Geometry: final body of the model. Coordinates: model frame, mm. Face numbers are marked on the shaded views. A direction names the side the tool comes from. Give positions to 0.01 mm unless a question says otherwise; leave off trailing zeros. Order: outer loops, then holes, each group sorted by start corner. A loop starts at its lowest first (then second) coordinate and runs counter-clockwise, first axis right, second up. Notation, with made-up numbers: (58.5, 21.25) - (83.5, 21.25) arc R19 ccw to (83.5, 57.25) - close; hole circle Ø5 at (66, -21). An arc over 180 degrees is marked (long way). Use one line per item in the form item = value.
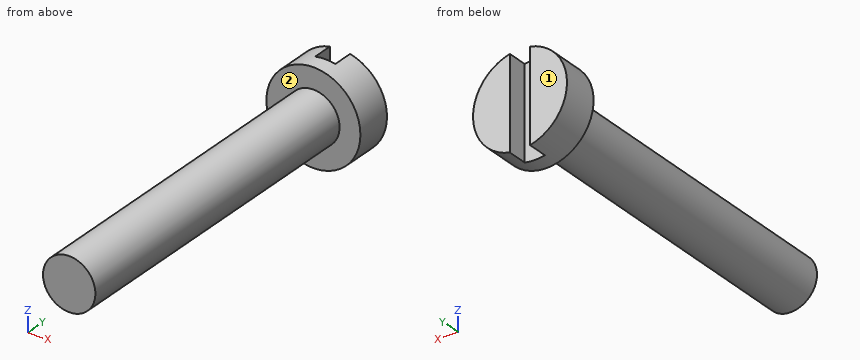
Autodesk Inventor part; units mm, degrees
ref_plane "YZ Plane" through (0, 0, 0) normal (1, 0, 0) x (0, 1, 0)
ref_plane "XZ Plane" through (0, 0, 0) normal (0, 1, 0) x (-1, 0, 0)
ref_plane "XY Plane" through (0, 0, 0) normal (0, 0, 1) x (1, 0, 0)
sketch "Sketch1" plane through (0, 0, 0) normal (0, 1, 0) x (-1, 0, 0)
  circle A0 centre (0, 0) radius 1.95
  dimension "d0" = 3.9
extrude "Extrusion1" add sketch "Sketch1" along normal blind 24.8
sketch "Sketch2" plane through (0, 24.8, 0) normal (0, 1, 0) x (1, 0, 0)
  circle A0 centre (0, 0) radius 3.5
  dimension "d3" = 7
extrude "Extrusion2" add sketch "Sketch2" along normal blind 2.7
sketch "Sketch3" plane through (0, 27.5, 0) normal (0, 1, 0) x (1, 0, 0)
  line L0 (0.75, -8) -> (-0.75, -8)
  line L1 (-0.75, -8) -> (-0.75, 8)
  line L2 (-0.75, 8) -> (0.75, 8)
  line L3 (0.75, 8) -> (0.75, -8)
  line L4 (0.75, -8) -> (-0.75, 8) construction
  line L5 (-0.75, -8) -> (0.75, 8) construction
  point P0 (0, 0)
  dimension "d6" = 1.5
  dimension "d7" = 16
extrude "Extrusion3" cut sketch "Sketch3" against normal blind 1.5
properties part number "screw27x4mm" material "Stainless Steel"
(1) Cut plane C-C on y = 20. Output: boundary loops of the cut face in (x, z), plus the area to 3 significant figures.
Computed values:
outline = circle Ø3.9 at (0, 0)
area = 11.9 mm²
(2) Contact query for flat-ended pins moving along their axis: pin 1 Ø3 at (x, z) = (0.5, 3) entering from +Y; pin 2 Ø1 at (x, y) = (-1, 18.5) entering from -Z; pin 3 Ø1.5 at (y, z) = (18, -2) entering from +X; pin 4 Ø4 at (y, z) = (5, 0.5) entering from -X. Output: stop coordinate, or through.
Computed values:
pin_1 = 27.5
pin_2 = -1.88
pin_3 = 1.5
pin_4 = -1.95
(3) Cut plane B-B on x = 0. Output: boundary loops of the cut face in (y, z), plus the area to 3 significant figures.
Computed values:
outline = (0, -1.95) - (24.8, -1.95) - (24.8, -3.5) - (26, -3.5) - (26, 3.5) - (24.8, 3.5) - (24.8, 1.95) - (0, 1.95) - close
area = 105 mm²
(4) Reachability of the marked faces 1 and 2 from +Z, -Z, +X, -X, +Y, -Y: full face, straight path, thin tool, end or side. Return the list, or none.
Computed values:
face_1 = +Z, -Z, +X, -X, +Y
face_2 = -Y
(5) Cut plane D-D on z = 2.5. Output: boundary loops of the cut face in (x, y).
Computed values:
outline = (-2.45, 24.8) - (2.45, 24.8) - (2.45, 27.5) - (0.75, 27.5) - (0.75, 26) - (-0.75, 26) - (-0.75, 27.5) - (-2.45, 27.5) - close
(6) Ray query, line 1 along Z through (x, y) = (0, 7.75); line 2 along Y through (x, z) = (-1.5, 2.5); line 3 along Y through (x, z) = (-0.5, 1.5). Return the intervals inside material, ascending.
Computed values:
line_1 = -1.95 to 1.95
line_2 = 24.8 to 27.5
line_3 = 0 to 26
(7) Cut plane A-A on z = 0. Output: boundary loops of the cut face in (x, y).
Computed values:
outline = (-3.5, 24.8) - (-1.95, 24.8) - (-1.95, 0) - (1.95, 0) - (1.95, 24.8) - (3.5, 24.8) - (3.5, 27.5) - (0.75, 27.5) - (0.75, 26) - (-0.75, 26) - (-0.75, 27.5) - (-3.5, 27.5) - close
